```python
from build123d import *

# Parameters (mm, degrees)
F1_DEPTH      = 40
F1_TAPER      = -20
F1_DEPTH_BACK = 20
F2_R          = 24.9048411139
F3_DEPTH      = 95
F3_TAPER      = 3


with BuildPart() as f1:
    # F0 (on Top) → F1 (new body, two sides)
    with BuildSketch(Plane.XY) as f1_sk:
        Polygon((-2.332799099, -41.0736999903), (38.3425354581, -14.9110951032), (26.029789227, 31.8581364071), (-22.2552409959, 34.600506221), (-39.7842845902, -10.4738475346), align=None)
    extrude(amount=-F1_DEPTH, taper=F1_TAPER)
    extrude(f1_sk.sketch, amount=F1_DEPTH_BACK)

    # F2 (on Top) → F3 (join)
    with BuildSketch(Plane.XY):
        Circle(F2_R)
    extrude(amount=F3_DEPTH, taper=F3_TAPER)


solid = f1.part
```
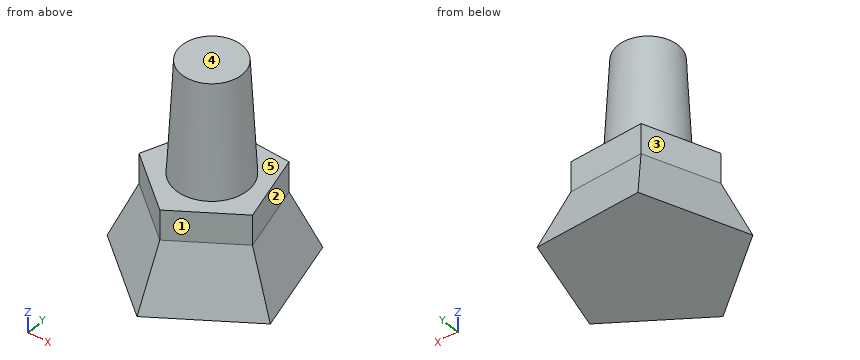
CAD build for the part. Positions are in the model's coordinates, mm. Face numbers are marked on the shaded views. A direction names the side the tool comes from. Round coordinates to 2 decimals unless told otherwise and drop trailing zeros. Order: outer loops, then holes, each group sorted by start corner. A loop starts at its lowest first (then second) coordinate and runs counter-clockwise, first axis right, second up. Notation, with made-up numbers: (-8.75, 67) - (29.25, 67) arc R30 ccw to (29.25, 93) - close; hole circle Ø11 at (65.25, 81.25). An arc over 180 degrees is marked (long way). Answer in a Markdown table with one row per item. Add a question column.
(1) Drop flat-ended pins along their axis: pin 1 Ø3 at (x, z) = (0, 80) entering from -Y; pin 2 Ø12 at (x, z) = (9.5, -20) entering from +Y; pin 3 Ø8 at (x, z) = (0, 70.5) entering from +Y. Give the stop position or say it passes through.
(2) Band-saw the part on A-A on z = 42.5. List the corners of the cut face in (x, y), and give its area (3 significant figures).
(3) Probe L1, parallel to Z at x = 28.5, y = -3; L2, parallel to X at y = 13.5, z = 31; L3, parallel to X at y = 32, z = -5.5. List the from-to ranges inside material, lowest first. Write a range as [from, to].
(4) 3-axis set-ups, long thin cutter, end or side, ignore diameter. For the marked faces 1, 2, 3, 4 and 5: which of +Z, -Z, +X, -X, +Y, -Y reach the whole face in a straight line?
Data:
| question | item | result |
|---|---|---|
| 1 | pin 1 | stops at y = -20.79 |
| 1 | pin 2 | stops at y = 42.3 |
| 1 | pin 3 | stops at y = 21.42 |
| 2 | outline | circle Ø45.36 at (0, 0) |
| 2 | area | 1,620 mm^2 |
| 3 | L1 | z = [-40, 20] |
| 3 | L2 | x = [-18.97, 18.97] |
| 3 | L3 | x = [-25.41, 28.06] |
| 4 | face 1 | +Z, +X, -Y |
| 4 | face 2 | +Z, +X, +Y |
| 4 | face 3 | +Z, -X, +Y |
| 4 | face 4 | +Z, +X, -X, +Y, -Y |
| 4 | face 5 | +Z |
